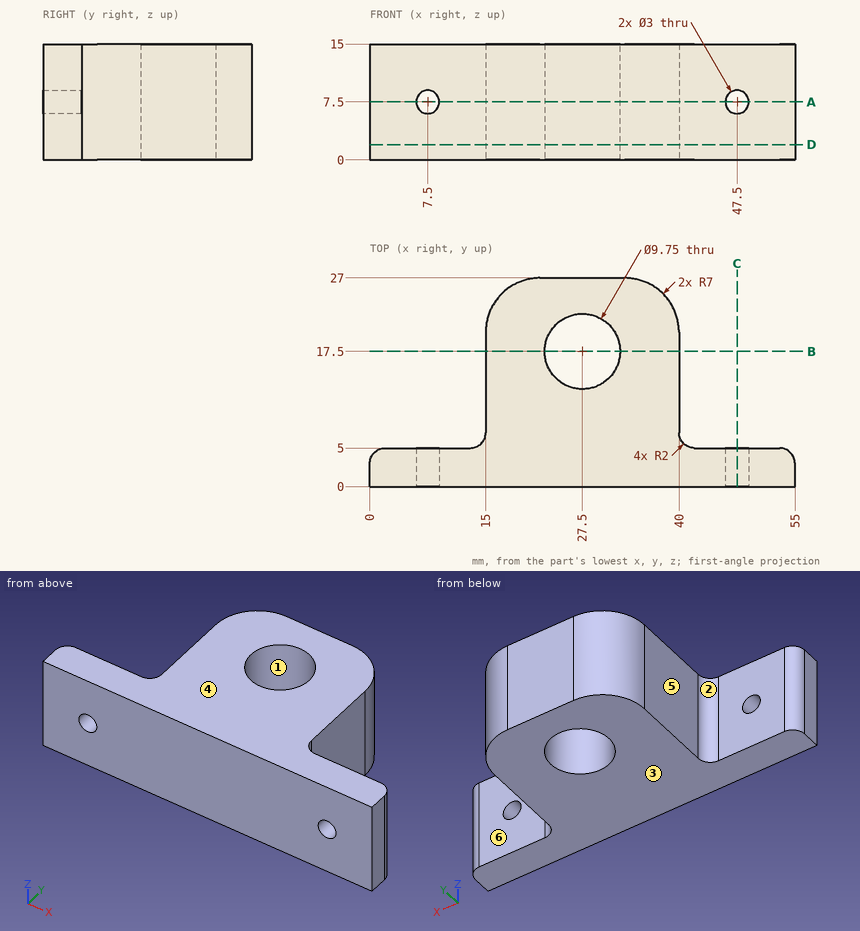
The drawing under review shows one solid part. Ordinate dimensions are in mm from its lowest x, y, z. A direction names the side the tool comes from. Coordinates: 2 decimals unless noted, no trailing zeros. Order: outer loops, then holes, each group sorted by start corner. A loop starts at its lowest first (then second) coordinate and runs counter-clockwise, first axis right, second up. Notation, with made-up numbers: (77, 20.5) -> (105, 20.5) arc R36 ccw to (105, 56.5) -> close; hole circle Ø11 at (1, 78). An arc over 180 degrees is marked (long way). Return JSON: item names as keys, results as strings.
1. We need section D-D on z = 2. Write out the cut boundary in (x, y) (3 decimals).
Answer block:
{"outline": "(0, 0) -> (55, 0) -> (55, 3) arc R2 ccw to (53, 5) -> (42, 5) arc R2 cw to (40, 7) -> (40, 20) arc R7 ccw to (33, 27) -> (22, 27) arc R7 ccw to (15, 20) -> (15, 7) arc R2 cw to (13, 5) -> (2, 5) arc R2 ccw to (0, 3) -> close; hole circle Ø9.75 at (27.5, 17.5)"}
2. For line 1 (Y direction, x = 27.5, z = 8) (3 decimals); line 2 (Z direction, x = 47.5, y = 3.65); line 3 (Y direction, x = 52, z = 9), list the stretches that pass through material, from the lowest coordinate up. Write a range as from..to.
Answer block:
{"line 1": "0..12.625, 22.375..27", "line 2": "0..6, 9..15", "line 3": "0..5"}
3. Machinability: for the marked faces 4, 5 and 6, which of the approach directions +Z, -Z, +X, -X, +Y, -Y give a long, thin tool a straight path to every point of the face, cutting with its end or side? Answer none if there is none.
Answer block:
{"face 4": "+Z, +X, -X, +Y, -Y", "face 5": "+Z, -Z, -X, +Y", "face 6": "+Z, -Z, +X, +Y"}
4. We need section C-C on x = 47.5. Write out the cut boundary in (y, z), and give its area (3 significant figures).
Answer block:
{"outline": "(0, 0) -> (5, 0) -> (5, 6) -> (0, 6) -> close; (0, 9) -> (5, 9) -> (5, 15) -> (0, 15) -> close", "area": "60.0 mm²"}
5. For pin 1 Ø12 at (x, y) = (28, 7.5) entering from -Z; pin 2 Ø5 at (y, z) = (16.5, 10.5) entering from +X; pin 3 Ø6 at (y, z) = (9.5, 13.5) entering from +X; pin 4 Ø9 at (x, z) = (50, 10.5) entering from +Y, all flat-tipped, find the tip position at first contact; note any pin that passes through.
Answer block:
{"pin 1": "z = 0", "pin 2": "x = 40", "pin 3": "x = 40.06", "pin 4": "y = 5"}
6. We need section A-A on z = 7.5. Write out the cut boundary in (x, y) (3 decimals).
Answer block:
{"outline": "(0, 0) -> (6, 0) -> (6, 5) -> (2, 5) arc R2 ccw to (0, 3) -> close; (9, 0) -> (46, 0) -> (46, 5) -> (42, 5) arc R2 cw to (40, 7) -> (40, 20) arc R7 ccw to (33, 27) -> (22, 27) arc R7 ccw to (15, 20) -> (15, 7) arc R2 cw to (13, 5) -> (9, 5) -> close; (49, 0) -> (55, 0) -> (55, 3) arc R2 ccw to (53, 5) -> (49, 5) -> close; hole circle Ø9.75 at (27.5, 17.5)"}
7. The part is to be moulded in two halves that separate along Y. For the marked faces 1, 2 and 3, say which applies: +Y half, -Y half, draft (parallel to the pull), parting line (faces both ways), or undercut.
Answer block:
{"face 1": "undercut", "face 2": "+Y half", "face 3": "draft"}
8. We need section B-B on y = 17.5. Write out the cut boundary in (x, z) (3 decimals).
Answer block:
{"outline": "(15, 0) -> (22.625, 0) -> (22.625, 15) -> (15, 15) -> close; (32.375, 0) -> (40, 0) -> (40, 15) -> (32.375, 15) -> close"}
